```python
from build123d import *

# Parameters (mm, degrees)
F0_W     = 1244.6
F0_H     = 28.575
F1_DEPTH = 220.6625
F3_DEPTH = 50.8
F4_DEPTH = 50.8


with BuildPart() as f1:
    # F0 (on Front) → F1 (new body, symmetric)
    with BuildSketch(Plane.XZ):
        Rectangle(F0_W, F0_H)
    extrude(amount=F1_DEPTH, both=True)

    # F2 (on face) → F3 (cut)
    with BuildSketch(Plane.XY.offset(14.2875)):
        with BuildLine():
            ThreePointArc((-438.683658, 139.539675), (-432.254002, 133.270344), (-425.98467, 139.7))
            Line((-425.98467, 139.7), (-425.985175, 202.879553))
            ThreePointArc((-425.985175, 202.879553), (-432.254609, 209.309109), (-438.684165, 203.039675))
            Line((-438.684165, 203.039675), (-438.683658, 139.539675))
        make_face()
        with BuildLine():
            ThreePointArc((-425.98467, -139.7), (-432.254002, -133.270344), (-438.683658, -139.539675))
            Line((-438.683658, -139.539675), (-438.684165, -203.039675))
            ThreePointArc((-438.684165, -203.039675), (-432.254609, -209.309109), (-425.985175, -202.879553))
            Line((-425.985175, -202.879553), (-425.98467, -139.7))
        make_face()
        with BuildLine():
            ThreePointArc((425.98467, 139.7), (432.254002, 133.270344), (438.683658, 139.539675))
            Line((438.683658, 139.539675), (438.684165, 203.039675))
            ThreePointArc((438.684165, 203.039675), (432.254609, 209.309109), (425.985175, 202.879553))
            Line((425.985175, 202.879553), (425.98467, 139.7))
        make_face()
        with BuildLine():
            Line((438.684165, -203.039675), (438.683658, -139.539675))
            ThreePointArc((438.683658, -139.539675), (432.254002, -133.270344), (425.98467, -139.7))
            Line((425.98467, -139.7), (425.985175, -202.879553))
            ThreePointArc((425.985175, -202.879553), (432.254609, -209.309109), (438.684165, -203.039675))
        make_face()
    extrude(amount=-F3_DEPTH, mode=Mode.SUBTRACT)

    # F2 (on face) → F4 (cut)
    with BuildSketch(Plane.XY.offset(14.2875)):
        with BuildLine():
            ThreePointArc((-558.8, -220.6625), (-606.109285, -114.808742), (-622.3, 0))
            Line((-622.3, 0), (-622.3, -220.6625))
            Line((-622.3, -220.6625), (-558.8, -220.6625))
        make_face()
        with BuildLine():
            Line((-622.3, 6.35), (-622.251434, 6.35))
            ThreePointArc((-622.251434, 6.35), (-605.219554, 117.85665), (-558.8, 220.6625))
            Line((-558.8, 220.6625), (-622.3, 220.6625))
            Line((-622.3, 220.6625), (-622.3, 6.35))
        make_face()
        with BuildLine():
            Line((622.3, -220.6625), (622.3, 0))
            ThreePointArc((622.3, 0), (606.109285, -114.808742), (558.8, -220.6625))
            Line((558.8, -220.6625), (622.3, -220.6625))
        make_face()
        with BuildLine():
            Line((622.251434, 6.35), (622.3, 6.35))
            Line((622.3, 6.35), (622.3, 220.6625))
            Line((622.3, 220.6625), (558.8, 220.6625))
            ThreePointArc((558.8, 220.6625), (605.219554, 117.85665), (622.251434, 6.35))
        make_face()
    extrude(amount=-F4_DEPTH, mode=Mode.SUBTRACT)


solid = f1.part
```
Design review of the part built by this model. Coordinates are the model's own, in mm. Give positions to 0.01 mm unless a question says otherwise; leave off trailing zeros. Write each loop counter-clockwise with the first axis right and the second up, starting at its lowest first coordinate (ties: lowest second). Pieces come first, ordered by that corner, then holes.
(1) Wall thickness on line 1 along X through (y, z) = (138.5, 12.5); line 2 along X through (y, z) = (-179, -1); line 3 along X through (y, z) = (8, -2): over which ranges is each line inside the solid? List them lowest first.
Checked values:
line 1: x = -598.52 to -438.58, -426.08 to 426.08, 438.58 to 598.52
line 2: x = -581.73 to -438.68, -425.98 to 425.98, 438.68 to 581.73
line 3: x = -622.22 to 622.22
(2) Add section A-A (z = 8.75). Give the boundary of the cut face in (x, y), and give its area (3 significant figures).
Checked values:
outline: (-622.3, 0) arc R415.15 ccw to (-558.8, -220.66) - (558.8, -220.66) arc R415.15 ccw to (622.3, 0) - (622.3, 6.35) - (622.25, 6.35) arc R415.15 ccw to (558.8, 220.66) - (-558.8, 220.66) arc R415.15 ccw to (-622.25, 6.35) - (-622.3, 6.35) - close; hole (-438.68, -203.04) arc R6.35 ccw to (-425.99, -202.88) - (-425.98, -139.7) arc R6.35 ccw to (-438.68, -139.54) - close; hole (-438.68, 139.54) arc R6.35 ccw to (-425.98, 139.7) - (-425.99, 202.88) arc R6.35 ccw to (-438.68, 203.04) - close; hole (425.98, -139.7) - (425.99, -202.88) arc R6.35 ccw to (438.68, -203.04) - (438.68, -139.54) arc R6.35 ccw to start; hole (425.98, 139.7) arc R6.35 ccw to (438.68, 139.54) - (438.68, 203.04) arc R6.35 ccw to (425.99, 202.88) - close
area: 527,000 mm2
(3) Add section B-B (y = 191). Give the boundary of the cut face in (x, z), and give its area (3 significant figures).
Checked values:
outline: (-575.75, -14.29) - (-438.68, -14.29) - (-438.68, 14.29) - (-575.75, 14.29) - close; (-425.99, -14.29) - (425.99, -14.29) - (425.99, 14.29) - (-425.99, 14.29) - close; (438.68, -14.29) - (575.75, -14.29) - (575.75, 14.29) - (438.68, 14.29) - close
area: 32,200 mm2
(4) Clearance check with flat-ended pins moving along their axes: pin 1 Ø14.5 at (y, z) = (-159.5, 1) entering from -X; pin 2 Ø14.5 at (y, z) = (-173, -1.5) entering from +X; pin 3 Ø1.5 at (y, z) = (-23, -8.5) entering from -X. State where each tip first meets the part, or that it passes through.
Checked values:
pin 1: stops at x = -593.37
pin 2: stops at x = 587.78
pin 3: stops at x = -621.7
